```python
from build123d import *

# Parameters (mm, degrees)
SKETCH1_R            = 41
BOSS_EXTRUDE1_DEPTH  = 1
SKETCH6_W            = 3
SKETCH6_H            = 41
BOSS_EXTRUDE7_DEPTH  = 25
SKETCH7_R            = 6
BOSS_EXTRUDE8_DEPTH  = 24
SKETCH9_R            = 6
CUT_EXTRUDE3_DEPTH   = 5
CIRPATTERN1_COUNT    = 8
SKETCH11_R           = 6
CUT_EXTRUDE5_DEPTH   = 6
BOSS_EXTRUDE9_DEPTH  = 2
CIRPATTERN2_COUNT    = 8
FILLET1_R            = 1
SKETCH13_R           = 6.5
BOSS_EXTRUDE17_DEPTH = 6
SKETCH16_R           = 6.5
SKETCH16_R_2         = 6
BOSS_EXTRUDE18_DEPTH = 24
SKETCH15_R           = 6
BOSS_EXTRUDE19_DEPTH = 3
SKETCH17_R           = 3.075
CUT_EXTRUDE10_DEPTH  = 5


with BuildPart() as part:
    # Sketch1 → Boss-Extrude1 (new body)
    with BuildSketch(Plane(origin=(0, 0, 0), x_dir=(1, 0, 0), z_dir=(0, 1, 0))):
        Circle(SKETCH1_R)
    extrude(amount=BOSS_EXTRUDE1_DEPTH)

    # Sketch6 → Boss-Extrude7 (add)
    with BuildSketch(Plane(origin=(0, 1, 0), x_dir=(1, 0, 0), z_dir=(0, 1, 0))):
        with Locations((0, -20.5)):
            Rectangle(SKETCH6_W, SKETCH6_H)
    boss_extrude7 = extrude(amount=BOSS_EXTRUDE7_DEPTH)

    # Sketch7 → Boss-Extrude8 (add)
    with BuildSketch(Plane.XZ):
        Circle(SKETCH7_R)
    extrude(amount=-BOSS_EXTRUDE8_DEPTH)

    # Sketch9 → Cut-Extrude3 (cut)
    with BuildSketch(Plane(origin=(0, 26, 0), x_dir=(1, 0, 0), z_dir=(0, 1, 0))):
        Circle(SKETCH9_R)
    extrude(amount=-CUT_EXTRUDE3_DEPTH, mode=Mode.SUBTRACT)

    # CirPattern1: Boss-Extrude7 ×8 about axis
    cirpattern1_axis = Axis((0, 0, 0), (0, 1, 0))
    for i in range(1, CIRPATTERN1_COUNT):
        add(boss_extrude7.rotate(cirpattern1_axis, i * 360 / CIRPATTERN1_COUNT))

    # Sketch11 → Cut-Extrude5 (cut)
    with BuildSketch(Plane(origin=(0, 26, 0), x_dir=(1, 0, 0), z_dir=(0, 1, 0))):
        Circle(SKETCH11_R)
    extrude(amount=-CUT_EXTRUDE5_DEPTH, mode=Mode.SUBTRACT)

    # Sketch10 → Boss-Extrude9 (add)
    with BuildSketch(Plane(origin=(0, 0, 0), x_dir=(-1, 0, 0), z_dir=(0, -1, 0))):
        Polygon((-3.142992858, 11.677824964), (-5.920826915, 10.544847493), (-7.809122701, 15.174570921), (-5.031288644, 16.307548393), align=None)
    boss_extrude9 = extrude(amount=BOSS_EXTRUDE9_DEPTH)

    # CirPattern2: Boss-Extrude9 ×8 about axis
    cirpattern2_axis = Axis((0, 0, 0), (0, 1, 0))
    for i in range(1, CIRPATTERN2_COUNT):
        add(boss_extrude9.rotate(cirpattern2_axis, i * 360 / CIRPATTERN2_COUNT))

    # Fillet1
    fillet1_edges = [part.edges().sort_by_distance(p)[0] for p in [
        (4.087140751, -2, -13.992686678),
        (6.420205673, -2, -15.741059657),
        (6.864974808, -2, -12.859709207),
        (4.531909887, -2, -11.111336228),
        (-7.004278697, -2, -12.784368578),
        (-6.590839059, -2, -15.670380994),
        (-4.238917345, -2, -13.947457824),
        (-4.652356983, -2, -11.061445408),
        (-13.992686678, -2, -4.087140751),
        (-15.741059657, -2, -6.420205673),
        (-12.859709207, -2, -6.864974808),
        (-11.111336228, -2, -4.531909887),
        (-12.784368578, -2, 7.004278697),
        (-15.670380994, -2, 6.590839059),
        (-13.947457824, -2, 4.238917345),
        (-11.061445408, -2, 4.652356983),
        (-4.087140751, -2, 13.992686678),
        (-6.420205673, -2, 15.741059657),
        (-6.864974808, -2, 12.859709207),
        (-4.531909887, -2, 11.111336228),
        (7.004278697, -2, 12.784368578),
        (6.590839059, -2, 15.670380994),
        (4.238917345, -2, 13.947457824),
        (4.652356983, -2, 11.061445408),
        (13.992686678, -2, 4.087140751),
        (15.741059657, -2, 6.420205673),
        (12.859709207, -2, 6.864974808),
        (11.111336228, -2, 4.531909887),
        (12.784368578, -2, -7.004278697),
        (15.670380994, -2, -6.590839059),
        (13.947457824, -2, -4.238917345),
        (11.061445408, -2, -4.652356983),
    ]]
    fillet(fillet1_edges, radius=FILLET1_R)

    # Sketch13 → Boss-Extrude17 (add)
    with BuildSketch(Plane(origin=(0, 20, 0), x_dir=(1, 0, 0), z_dir=(0, 1, 0))):
        Circle(SKETCH13_R)
    extrude(amount=BOSS_EXTRUDE17_DEPTH)

    # Sketch16 → Boss-Extrude18 (add)
    with BuildSketch(Plane(origin=(0, 26, 0), x_dir=(1, 0, 0), z_dir=(0, 1, 0))):
        Circle(SKETCH16_R)
        Circle(SKETCH16_R_2, mode=Mode.SUBTRACT)
    extrude(amount=-BOSS_EXTRUDE18_DEPTH)

    # Sketch15 → Boss-Extrude19 (add)
    with BuildSketch(Plane.XZ):
        Circle(SKETCH15_R)
    extrude(amount=BOSS_EXTRUDE19_DEPTH)

    # Sketch17 → Cut-Extrude10 (cut)
    with BuildSketch(Plane.XZ.offset(3)):
        Circle(SKETCH17_R)
    extrude(amount=-CUT_EXTRUDE10_DEPTH, mode=Mode.SUBTRACT)


solid = part.part
```
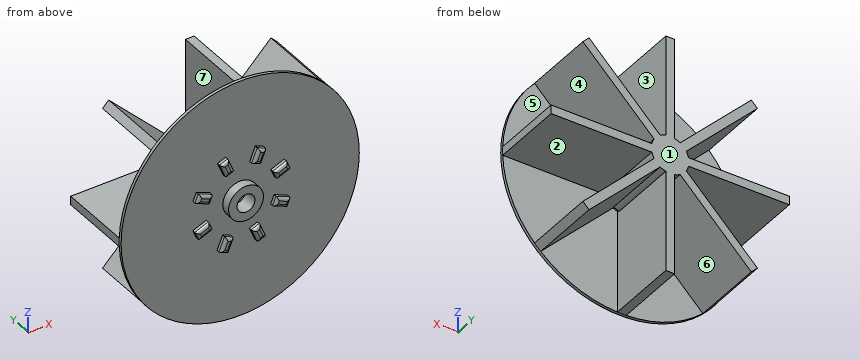
Geometry check sheet. Reference: the model listing, model coordinates, mm. Face numbers are marked on the shaded views. A direction names the side the tool comes from. Round coordinates to 2 decimals unless told otherwise and drop trailing zeros. Loops run counter-clockwise (first coordinate to the right, second up) from the corner with the lowest first, then second, coordinate; pieces in that order, holes last. Notation, with made-up numbers: M 57.5,-12 L 97.5,-12 A28 cw 97.5,16 Z; hole C 76,26 d11. An arc over 180 degrees is marked long. Return JSON: item names as keys, results as strings. Group by question number.
(1) Set-up check for the marked faces 1, 2 and 3: record each of +Z, -Z, +X, -X, +Y, -Y from which the full face is reachable in a straight line by a thin tool's end or side.
(2) Go/stop test with flat-tipped pins: pin 1 (2.5 mm diameter, centred on x = 14, z = 5, fed in from -Y); pin 2 (1 mm diameter, centred on y = 12, z = 28, fed in from +X); pin 3 (4 mm diameter, centred on y = 14.5, z = 6.5, fed in from -X); pin 4 (0.5 mm diameter, centred on x = 28.5, z = 30, fed in from -Y). Record where each tip stops, or that it passes through.
(3) Scan lines: line 1 along Z through (x, y) = (0, 0.2) (3 decimals); line 2 along Z through (x, y) = (0, -0.25) (3 decimals); line 3 along X through (y, z) = (17.5, -21). Record each from-to range of solid material in increasing order. Write a range as [from, to].
(4) Section check D-D, the plane x = -33.5. Enter the section's corners in (y, z), and give its area (3 significant figures).
(5) Mould release check, pull along Z, two halves, no side actions. Record for the marked faces 4, 5, 6 and 7: pulls with the +Z half, pulls with the -Z half, needs draft (parallel to the pull), parting line crosses it, or undercut.
(6) Section check C-C, the plane z = -20. Enter the section's corners in (x, y), and give its area (3 significant figures).
(7) Section check A-A, the plane x = -17.5. Enter the section's corners in (y, z).
Data:
{
 "1": {"face 1": "+Z, -Z, +X, -X, +Y", "face 2": "+X, +Y", "face 3": "+Z, +Y"},
 "2": {"pin 1": "y = -2", "pin 2": "x = 30.05", "pin 3": "x = -10.62", "pin 4": "through"},
 "3": {"line 1": "[-41, -3.075], [3.075, 41]", "line 2": "[-6, -3.075], [3.075, 6]", "line 3": "[-23.12, -18.88], [-1.5, 1.5], [18.88, 23.12]"},
 "4": {"outline": "M 0,-23.64 L 1,-23.64 L 1,-1.5 L 26,-1.5 L 26,1.5 L 1,1.5 L 1,23.64 L 0,23.64 Z", "area": "122 mm²"},
 "5": {"face 4": "undercut", "face 5": "undercut", "face 6": "pulls with the -Z half", "face 7": "needs draft"},
 "6": {"outline": "M -35.79,0 L 35.79,0 L 35.79,1 L 22.12,1 L 22.12,26 L 17.88,26 L 17.88,1 L 1.5,1 L 1.5,26 L -1.5,26 L -1.5,1 L -17.88,1 L -17.88,26 L -22.12,26 L -22.12,1 L -35.79,1 Z", "area": "359 mm²"},
 "7": {"outline": "M 0,-37.08 L 1,-37.08 L 1,-19.62 L 26,-19.62 L 26,-15.38 L 1,-15.38 L 1,-1.5 L 26,-1.5 L 26,1.5 L 1,1.5 L 1,15.38 L 26,15.38 L 26,19.62 L 1,19.62 L 1,37.08 L 0,37.08 Z"}
}
